from build123d import *

# Parameters (mm, degrees)
F1_DEPTH  = 50.8
F2_T      = -3.175
F3_W      = 323.85
F3_H      = 361.95
F4_DEPTH  = 25.4
F5_W      = 47.625
F5_H      = 47.625
F6_DEPTH  = 254
F7_W      = 47.625
F7_H      = 47.625
F8_DEPTH  = 25.4
F10_DEPTH = 25.4


with BuildPart() as f1:
    # F0 (on Top) → F1 (new body)
    with BuildSketch(Plane.XY):
        Polygon((-298.1223497814, 269.3835347245), (-298.1223497814, 0), (-298.1223497814, -200.5164652755), (260.6776502186, -200.5164652755), (260.6776502186, -111.6164652755), (133.6776502186, -111.6164652755), (133.6776502186, 269.3835347245), align=None)
    extrude(amount=F1_DEPTH)

    # F2
    f2_openings = [f1.faces().sort_by_distance(p)[0] for p in [
        (-67.49494, 24.392119, 50.8),
    ]]
    offset(amount=F2_T, openings=f2_openings, kind=Kind.INTERSECTION)

    # F3 (on face) → F4 (cut)
    with BuildSketch(Plane.XY.offset(3.175)):
        with Locations((-82.2223497814, 34.4335347245)):
            Rectangle(F3_W, F3_H)
    extrude(amount=-F4_DEPTH, mode=Mode.SUBTRACT)

    # F5 (on face) → F6 (cut, symmetric)
    with BuildSketch(Plane.XZ.offset(-266.2085347245)):
        with Locations((-271.1348497814, 26.9875)):
            Rectangle(F5_W, F5_H)
    extrude(amount=F6_DEPTH, both=True, mode=Mode.SUBTRACT)

    # F7 (on face) → F8 (cut)
    with BuildSketch(Plane(origin=(0, -197.3414652755, 0), x_dir=(-1, 0, 0), z_dir=(0, 1, 0))):
        with Locations((271.1348497814, 26.9875)):
            Rectangle(F7_W, F7_H)
    extrude(amount=-F8_DEPTH, mode=Mode.SUBTRACT)

    # F9 (on face) → F10 (cut)
    with BuildSketch(Plane.XY.offset(3.175)):
        Polygon((130.5026502186, -162.4164652755), (130.5026502186, -114.7914652755), (79.7026502186, -114.7914652755), (79.7026502186, -197.3414652755), (257.5026502186, -197.3414652755), (257.5026502186, -162.4164652755), align=None)
    extrude(amount=-F10_DEPTH, mode=Mode.SUBTRACT)


solid = f1.part
For this review, take the finished solid that the model builds, in its own axes (mm). A direction names the side the tool comes from. Give positions to 0.01 mm unless a question says otherwise; leave off trailing zeros. Order: outer loops, then holes, each group sorted by start corner. A loop starts at its lowest first (then second) coordinate and runs counter-clockwise, first axis right, second up. Notation, with made-up numbers: (24.25, 46.25) -> (40.25, 46.25) arc R7 ccw to (40.25, 54.25) -> close; hole circle Ø3 at (32.5, 46). An arc over 180 degrees is marked (long way). Write item = value, one per line.
1) We need section A-A, the plane y = -170.5. Give the boundary of the cut face in (x, z) (3 decimals), and give its area (3 significant figures).
Findings:
outline = (-298.122, 0) -> (79.703, 0) -> (79.703, 3.175) -> (-294.947, 3.175) -> (-294.947, 50.8) -> (-298.122, 50.8) -> close; (257.503, 0) -> (260.678, 0) -> (260.678, 50.8) -> (257.503, 50.8) -> close
area = 1,510 mm^2
2) For faces 1 (the face through (257.503, -157, 26)), 2 (the face through (-298.122, 38, 25)), 3 (the face through (133.678, 76, 25)), list the 3-axis set-ups (+Z, -Z, +X, -X, +Y, -Y) from which the entire face can be reached by the end or side of a thin tool; tool diameter is ignored.
Findings:
face_1 = +Z
face_2 = +Z, -Z, -X, +Y, -Y
face_3 = +Z, -Z, +X, +Y
3) We need section B-B, the plane z = 36.5. Give the boundary of the cut face in (x, y), and give its area (3 significant figures).
Findings:
outline = (-298.12, -200.52) -> (-294.95, -200.52) -> (-294.95, 269.38) -> (-298.12, 269.38) -> close; (-247.32, -200.52) -> (260.68, -200.52) -> (260.68, -111.62) -> (133.68, -111.62) -> (133.68, 269.38) -> (-247.32, 269.38) -> (-247.32, 266.21) -> (130.5, 266.21) -> (130.5, -114.79) -> (257.5, -114.79) -> (257.5, -197.34) -> (-247.32, -197.34) -> close
area = 6,190 mm^2
4) Insertion check: pin 1 (4 mm diameter, centred on y = -16, z = 42.5, fed in from +X); pin 2 (4 mm diameter, centred on x = 198, y = -130, fed in from -Z); pin 3 (24 mm diameter, centred on x = 166.5, y = -127, fed in from +Z) (3 decimals). Each pin has a flat end and moves straight along its axis. Give the tip position at first contact, or say it passes through.
Findings:
pin_1 = 133.68
pin_2 = 0
pin_3 = 3.175
5) Draft analysis for pull direction X (two halves, no side actions). For faces 4 (the face through (-79, 269.384, 25)), 5 (the face through (260.678, -157, 25)), 6 (the face through (-294.947, 31, 27)), state which applies: pulls with the +X half, pulls with the -X half, needs draft (parallel to the pull), parting line crosses it, or undercut.
Findings:
face_4 = needs draft
face_5 = pulls with the +X half
face_6 = undercut
6) We need section D-D, the plane y = -95. Give the boundary of the cut face in (x, z) (3 decimals).
Findings:
outline = (-298.122, 0) -> (-244.147, 0) -> (-244.147, 3.175) -> (-294.947, 3.175) -> (-294.947, 50.8) -> (-298.122, 50.8) -> close; (79.703, 0) -> (133.678, 0) -> (133.678, 50.8) -> (130.503, 50.8) -> (130.503, 3.175) -> (79.703, 3.175) -> close
7) To check wall thickness, follow L1, parallel to Y at x = 69.5, z = 14; L2, parallel to X at y = -120, z = 18.5; L3, parallel to X at y = 241, z = 15.5. State the ranges of each line that lie inside material, in increasing order. Write a range as from..to.
Findings:
L1 = -200.52..-197.34, 266.21..269.38
L2 = -298.12..-294.95, 257.5..260.68
L3 = -298.12..-294.95, 130.5..133.68
8) We need section C-C, the plane x = -60.5. Give the boundary of the cut face in (y, z) (3 decimals).
Findings:
outline = (-200.516, 0) -> (-146.541, 0) -> (-146.541, 3.175) -> (-197.341, 3.175) -> (-197.341, 50.8) -> (-200.516, 50.8) -> close; (215.409, 0) -> (269.384, 0) -> (269.384, 50.8) -> (266.209, 50.8) -> (266.209, 3.175) -> (215.409, 3.175) -> close
